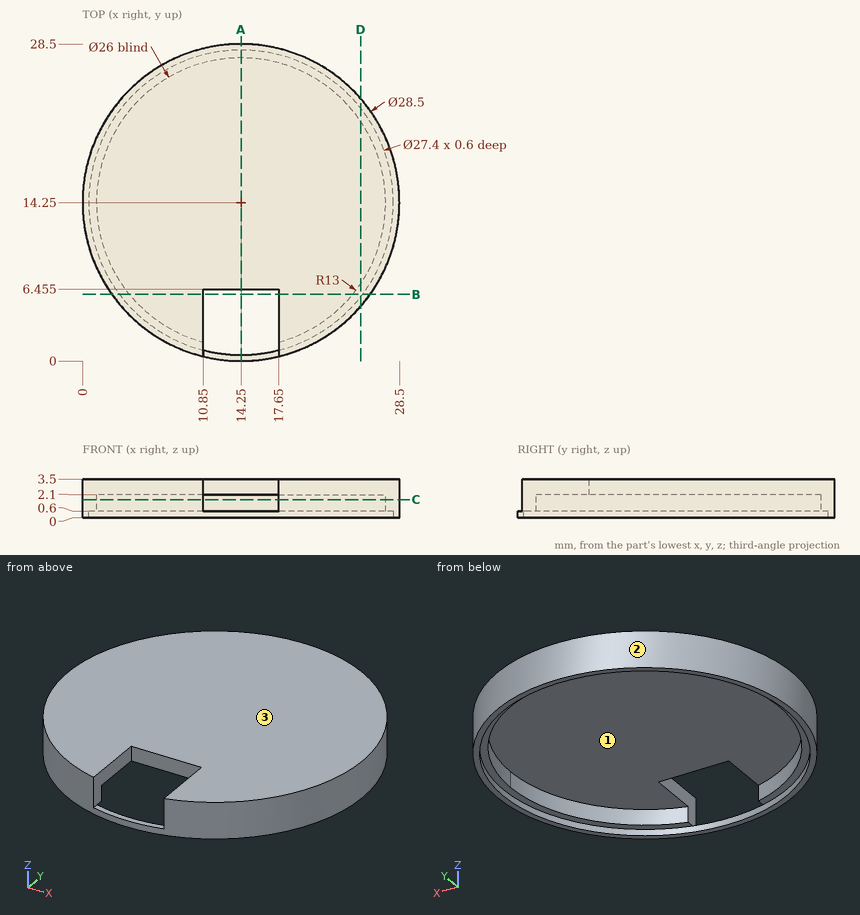
Can you work these out from the drawing? Everything is in mm from the part's minimum corner. Round coordinates to 2 decimals unless told otherwise and drop trailing zeros. Loops run counter-clockwise (first coordinate to the right, second up) from the corner with the lowest first, then second, coordinate; pieces in that order, holes last. Notation, with made-up numbers: (-19, -9) -> (24, -9) arc R28 cw to (24, 26) -> close; hole circle Ø6 at (-14.75, -10.5). An arc over 180 degrees is marked (long way). Answer in a Markdown table with one row per item.
Item 1: If I drill on probe 1 along X at (y, z) = (14.25, 0.2); probe 2 along X at (y, z) = (14.25, 1.45); probe 3 along Y at (x, z) = (24.75, 0.25), over which ranges is the centre line in solid material (lowest first)?
Answer block:
| item | result |
|---|---|
| probe 1 | 0 to 0.55, 27.95 to 28.5 |
| probe 2 | 0 to 1.25, 27.25 to 28.5 |
| probe 3 | 4.62 to 5.45, 23.05 to 23.88 |
Item 2: We'd pull the mould along Y, two halves only. Please class the marked faces 1, 2 and 3: released by +Y, released by -Y, zero draft, split by the parting line, or undercut.
Answer block:
| item | result |
|---|---|
| face 1 | undercut |
| face 2 | split by the parting line |
| face 3 | zero draft |
Item 3: Suppose I cut it at D-D, the plane x = 25. List the corners of the cut face in (y, z) for me, plus the area to 3 significant figures.
Answer block:
| item | result |
|---|---|
| outline | (4.9, 0) -> (5.76, 0) -> (5.76, 0.6) -> (6.94, 0.6) -> (6.94, 2.1) -> (21.56, 2.1) -> (21.56, 0.6) -> (22.74, 0.6) -> (22.74, 0) -> (23.6, 0) -> (23.6, 3.5) -> (4.9, 3.5) -> close |
| area | 33.4 mm² |
Item 4: Will these pins go through, and if not, where does the flat tip stop? P1, Ø1.1, axis at x = 14.5, z = 3, coming from the -Y side (3 decimals); P2, Ø4, axis at x = 15, y = 21.5, coming from the -Z side; P3, Ø1.1, axis at x = 12.5, y = 0.5, coming from the +Z side.
Answer block:
| item | result |
|---|---|
| P1 | y = 6.455 |
| P2 | z = 2.1 |
| P3 | z = 0.6 |
Item 5: Suppose I cut it at C-C, the plane z = 1.65. List the corners of the cut face in (x, y) for me, plus the area to 3 significant figures.
Answer block:
| item | result |
|---|---|
| outline | (10.85, 0.41) -> (10.85, 1.7) arc R13 cw (long way) to (17.65, 1.7) -> (17.65, 0.41) arc R14.25 ccw (long way) to start |
| area | 98.4 mm² |
Item 6: Suppose I cut it at A-A, the plane x = 14.25. List the corners of the cut face in (y, z) for me (3 decimals).
Answer block:
| item | result |
|---|---|
| outline | (0, 0) -> (0.55, 0) -> (0.55, 0.6) -> (0, 0.6) -> close; (6.455, 2.1) -> (27.25, 2.1) -> (27.25, 0.6) -> (27.95, 0.6) -> (27.95, 0) -> (28.5, 0) -> (28.5, 3.5) -> (6.455, 3.5) -> close |
Item 7: Suppose I cut it at B-B, the plane y = 6. List the corners of the cut face in (x, z) for me, plus the area to 3 significant figures.
Answer block:
| item | result |
|---|---|
| outline | (2.63, 0) -> (3.31, 0) -> (3.31, 0.6) -> (4.2, 0.6) -> (4.2, 2.1) -> (10.85, 2.1) -> (10.85, 3.5) -> (2.63, 3.5) -> close; (17.65, 2.1) -> (24.3, 2.1) -> (24.3, 0.6) -> (25.19, 0.6) -> (25.19, 0) -> (25.87, 0) -> (25.87, 3.5) -> (17.65, 3.5) -> close |
| area | 28.5 mm² |
